Print and shaded views of the part. All mm, measured from the part's lowest x, y and z. A direction names the side the tool comes from. Round coordinates to 2 decimals unless told otherwise and drop trailing zeros. Loops run counter-clockwise (first coordinate to the right, second up) from the corner with the lowest first, then second, coordinate; pieces in that order, holes last. Notation, with made-up numbers: (-31, 13.5) -> (-6, 13.5) arc R29 cw to (-6, 52.5) -> close; hole circle Ø3 at (87.25, 51). An arc over 180 degrees is marked (long way). Answer as CSV lines item,"result".
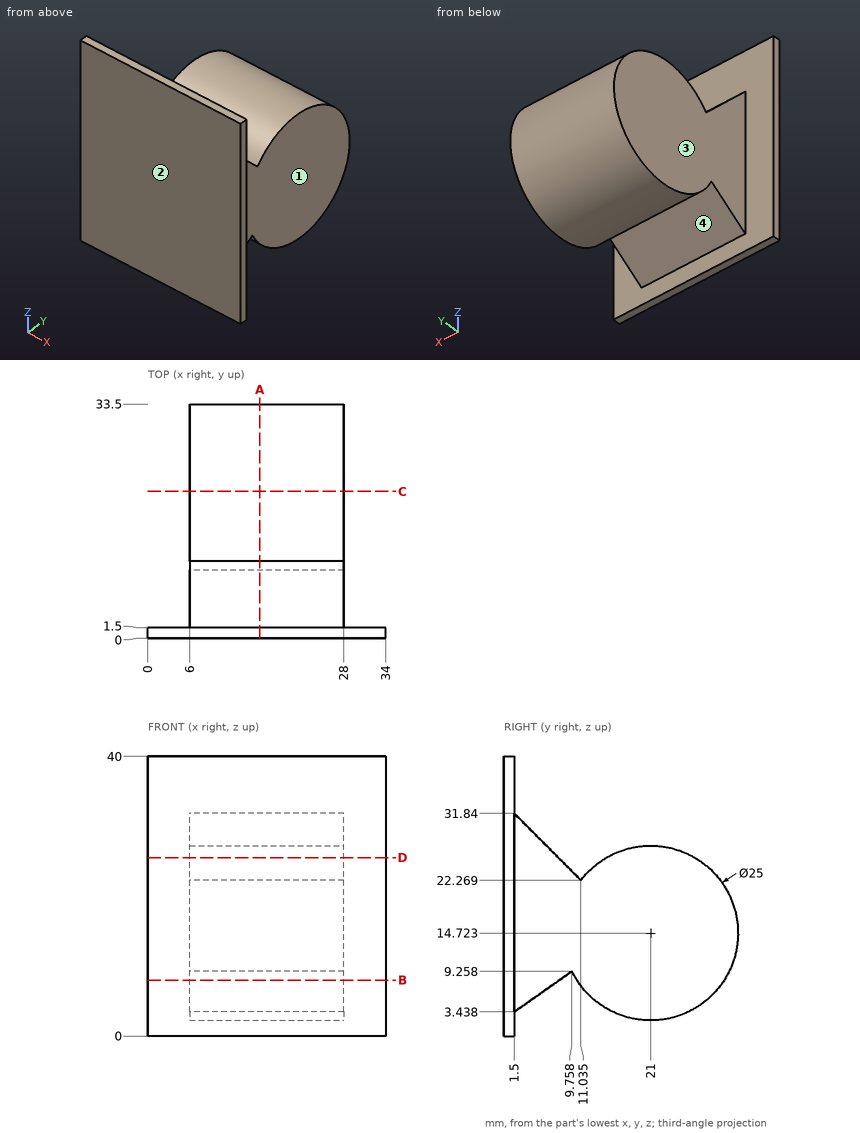
Q1. Tool access for the marked faces 1, 2, 3 and 4: list every direction of +Z, -Z, +X, -X, +Y, -Y with a clear straight run to the whole face (end or side of a thin tool).
Results:
face 1,"+Z, -Z, +X, +Y"
face 2,"+Z, -Z, +X, -X, -Y"
face 3,"+Z, -Z, -X, +Y"
face 4,"-Z, +X, -X"
Q2. Drop flat-ended pins along their axis: pin 1 Ø3 at (y, z) = (19.5, 22.5) entering from +X; pin 2 Ø2 at (y, z) = (8, 29.5) entering from +X; pin 3 Ø5 at (x, y) = (21, 24.5) entering from +Z; pin 4 Ø10 at (y, z) = (17.5, 19.5) entering from -X. Give the stop position or say it passes through.
Results:
pin 1,"x = 28"
pin 2,"through"
pin 3,"z = 27.18"
pin 4,"x = 6"
Q3. Slice it at B-B, the plane z = 8. Give the cut face in (x, y), and give its area (3 significant figures).
Results:
outline,"(0, 0) -> (34, 0) -> (34, 1.5) -> (28, 1.5) -> (28, 7.97) -> (6, 7.97) -> (6, 1.5) -> (0, 1.5) -> close; (6, 10.46) -> (28, 10.46) -> (28, 31.54) -> (6, 31.54) -> close"
area,"657 mm2"
Q4. Probe L1, parallel to X at y = 7, z = 16; L2, parallel to Y at x = 30, z = 19; L3, parallel to Y at x = 7, z = 8 (1 decimal). List the from-to ranges inside material, lowest first. Write a range as [from, to].
Results:
L1,"[6, 28]"
L2,"[0, 1.5]"
L3,"[0, 8], [10.5, 31.5]"
Q5. Slice it at A-A, the plane x = 16. Give the cut face in (y, z) (1 decimal).
Results:
outline,"(0, 0) -> (1.5, 0) -> (1.5, 3.4) -> (9.8, 9.3) arc R12.5 ccw (long way) to (11, 22.3) -> (1.5, 31.8) -> (1.5, 40) -> (0, 40) -> close"
Q6. Slice it at C-C, the plane y = 21. Give the cut face in (x, z).
Results:
outline,"(6, 2.22) -> (28, 2.22) -> (28, 27.22) -> (6, 27.22) -> close"
Q7. Slice it at D-D, the plane z = 25.5. Give the cut face in (x, y).
Results:
outline,"(0, 0) -> (34, 0) -> (34, 1.5) -> (28, 1.5) -> (28, 7.82) -> (6, 7.82) -> (6, 1.5) -> (0, 1.5) -> close; (6, 14.67) -> (28, 14.67) -> (28, 27.33) -> (6, 27.33) -> close"
